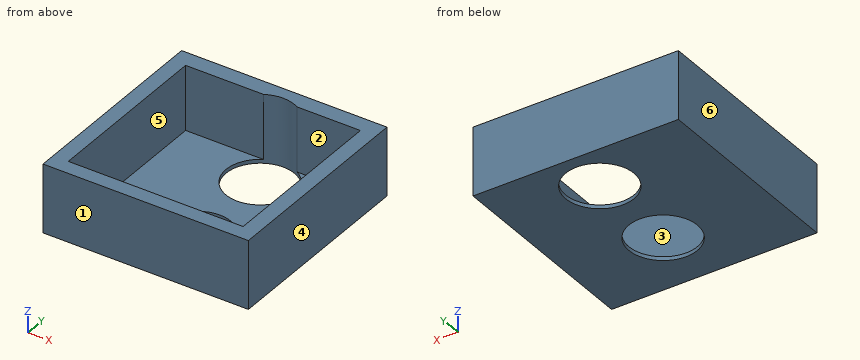
Autodesk Inventor part; units mm, degrees
ref_plane "YZ Plane" through (0, 0, 0) normal (1, 0, 0) x (0, 1, 0)
ref_plane "XZ Plane" through (0, 0, 0) normal (0, 1, 0) x (-1, 0, 0)
ref_plane "XY Plane" through (0, 0, 0) normal (0, 0, 1) x (1, 0, 0)
sketch "Sketch1" plane through (0, 0, 0) normal (0, 0, 1) x (1, 0, 0)
  line L0 (-15.4228, 9.2021) -> (98.8772, 9.2021)
  line L1 (98.8772, 9.2021) -> (98.8772, -105.0979)
  line L2 (98.8772, -105.0979) -> (-15.4228, -105.0979)
  line L3 (-15.4228, -105.0979) -> (-15.4228, 9.2021)
  point P0 (0, 0)
  dimension "d0" = 114.3
  dimension "d1" = 114.3
extrude "Extrusion1" add sketch "Sketch1" along normal blind 38.1
sketch "Sketch2" plane through (0, 0, 38.1) normal (0, 0, 1) x (1, 0, 0)
  line L0 (-6.9895, 0) -> (90.3039, 0)
  line L1 (90.3039, 0) -> (90.3039, -96.7342)
  line L2 (90.3039, -96.7342) -> (-6.9895, -96.7342)
  line L3 (-6.9895, -96.7342) -> (-6.9895, 0)
  point P0 (0, 0)
extrude "Extrusion2" cut sketch "Sketch2" against normal blind 36
sketch "Sketch3" plane through (0, 0, 0) normal (0, 0, -1) x (-1, 0, 0)
  circle A0 centre (-45.7039, -16.5922) radius 19.05
  circle A1 centre (-45.7039, -68.7821) radius 19.05
  point P0 (0, 0)
  dimension "d6" = 38.1
  dimension "d7" = 38.1
extrude "Extrusion3" cut sketch "Sketch3" against normal through all
properties part number "ledbox"
Build history of the part. All positions in model axes, mm. Face numbers are marked on the shaded views. A direction names the side the tool comes from. Round coordinates to 2 decimals unless told otherwise and drop trailing zeros. Loops run counter-clockwise (first coordinate to the right, second up) from the corner with the lowest first, then second, coordinate; pieces in that order, holes last. Notation, with made-up numbers: (21.5, 12.5) -> (39.5, 12.5) arc R24 cw to (39.5, 29.5) -> close; hole circle Ø11 at (-6, 57). An arc over 180 degrees is marked (long way). One line per item, written item: value. Start each with the question number.
Q1. Two-plate mould, pull along Y, no slides. Class the marked faces 1, 2, 3 and 4: released by +Y, released by -Y, zero draft, split by the parting line, or undercut.
Q2. Cut at D-D on x = 43. List the corners of the cut face in (y, z), plus the area to 3 significant figures.
Q3. 3-axis set-ups, long thin cutter, end or side, ignore diameter. For the marked faces 5 and 6: which of +Z, -Z, +X, -X, +Y, -Y reach the whole face in a straight line?
Q4. Drop flat-ended pins along their axis: pin 1 Ø12 at (x, y) = (82, -60.5) entering from +Z; pin 2 Ø1.5 at (x, y) = (70.5, -11) entering from -Z. Give the stop position or say it passes through.
Q5. Cut at A-A on x = 25. List the corners of the cut face in (y, z).
Q6. Cut at B-B on y = -19. List the corners of the cut face in (x, z), plus the area to 3 significant figures.
Q7. Probe line 1 along X through (y, z) = (-24, 23); line 2 along Y through (x, z) = (36, 33); line 3 along Z through (x, y) = (0.5, -61.5). List the from-to ranges inside material, lowest first.
Q8. Cut at C-C on z = 24. List the corners of the cut face in (x, y).
Computed:
1. face 1: released by -Y
1. face 2: undercut
1. face 3: undercut
1. face 4: zero draft
2. outline: (-105.1, 0) -> (-87.64, 0) -> (-87.64, 2.1) -> (-96.73, 2.1) -> (-96.73, 38.1) -> (-105.1, 38.1) -> close; (-49.92, 0) -> (-35.45, 0) -> (-35.45, 2.1) -> (-49.92, 2.1) -> close; (2.26, 0) -> (9.2, 0) -> (9.2, 38.1) -> (2.26, 38.1) -> close
2. area: 632 mm²
3. face 5: +Z
3. face 6: +Z, -Z, -X, +Y, -Y
4. pin 1: z = 2.1
4. pin 2: z = 0
5. outline: (-105.1, 0) -> (9.2, 0) -> (9.2, 38.1) -> (0, 38.1) -> (0, 2.1) -> (-96.73, 2.1) -> (-96.73, 38.1) -> (-105.1, 38.1) -> close
6. outline: (-15.42, 0) -> (26.81, 0) -> (26.81, 2.1) -> (-6.99, 2.1) -> (-6.99, 38.1) -> (-15.42, 38.1) -> close; (64.6, 0) -> (98.88, 0) -> (98.88, 38.1) -> (90.3, 38.1) -> (90.3, 2.1) -> (64.6, 2.1) -> close
6. area: 773 mm²
7. line 1: -15.42 to -6.99, 90.3 to 98.88
7. line 2: -105.1 to -96.73, 0 to 9.2
7. line 3: 0 to 2.1
8. outline: (-15.42, -105.1) -> (98.88, -105.1) -> (98.88, 9.2) -> (-15.42, 9.2) -> close; hole (-6.99, -96.73) -> (90.3, -96.73) -> (90.3, 0) -> (55.06, 0) arc R19.05 ccw to (36.34, 0) -> (-6.99, 0) -> close
